For this review, take the finished solid that the model builds, in its own axes (mm). A direction names the side the tool comes from. Coordinates: 2 decimals unless noted, no trailing zeros. Write each loop counter-clockwise with the first axis right and the second up, starting at its lowest first coordinate (ties: lowest second). Pieces come first, ordered by that corner, then holes. Notation, with made-up numbers: (-38, -25) -> (11, -25) arc R20 ccw to (11, 8) -> close; hole circle Ø11 at (56.5, 50). An arc over 180 degrees is marked (long way). Put each result on its own line as item: value. Start each with the question number.
Item 1: Insertion check: P1, Ø4, axis at x = -12.73, y = -30.38, coming from the +Z side; P2, Ø2, axis at x = -10.5, y = 22, coming from the +Z side; P3, Ø1, axis at y = 15.5, z = 10, coming from the +X side; P4, Ø9.5, axis at x = -2.5, y = -13, coming from the -Z side. Each pin has a flat end and moves straight along its axis. Give the tip position at first contact, or say it passes through.
Item 2: For faces 1 (the flat face through (-4, 22.359, 1)), 2 (the flat face through (-15, -30, 0)), 3 (the flat face through (7, -30, 0)), 4 (the cylindrical face through (12.01, -26.95, -1.52)), 5 (the cylindrical face through (-19.464, 22.929, -1.521)), list the 3-axis set-ups (+Z, -Z, +X, -X, +Y, -Y) from which the entire face can be reached by the end or side of a thin tool; tool diameter is ignored.
Item 3: Consider section D-D on y = -27. Give the boundary of the cut face in (x, z).
Item 4: Consider section B-B on x = 7.5. Give the boundary of the cut face in (y, z).
Item 5: To check wall thickness, follow L1, parallel to Y at x = -5.5, z = -1.5; L2, parallel to X at y = -29.5, z = 6; L3, parallel to Z at x = -9, y = -3. State the ranges of each line that lie inside material, in increasing order.
Item 6: Consider section C-C on z = -1.5. Give the boundary of the cut face in (x, y).
Item 7: Consider section A-A on z = 6. Give the boundary of the cut face in (x, y).
Item 8: The part is to be moulded in two halves that separate along Y. For faces 6 (the flat face through (-4, -2, 10)), 7 (the cylindrical face through (12.01, -33.81, -1.52)), 8 (the flat face through (-4, 26, -3)), say which applies: +Y half, -Y half, draft (parallel to the pull), parting line (faces both ways), or undercut.
```python
from build123d import *

# Parameters (mm, degrees)
SKETCH_1_W             = 32.677388302
SKETCH_1_H             = 8
EXTRUDE_1_DEPTH        = 3
SKETCH_2_R             = 1.5
CUT_EXTRUDE_1_DEPTH    = 4
SKETCH_3_R             = 6
EXTRUDE_2_DEPTH        = 8
EXTRUDE_3_DEPTH        = 8
SKETCH_10_W            = 12
SKETCH_10_H            = 24.37
EXTRUDE_5_DEPTH        = 2
SKETCH_4_R             = 4
CUT_EXTRUDE_2_DEPTH    = 9
FILLET_1_R             = 2
MIRROR_3_COPY_1_DEPTH  = 8
FILLET_1_OF_MIRROR_3_R = 2


with BuildPart() as part:
    # Sketch 1 → Extrude 1 (new body)
    with BuildSketch(Plane.XY):
        with Locations((-3.726697353, 26.358574689)):
            Rectangle(SKETCH_1_W, SKETCH_1_H)
    extrude_1 = extrude(amount=-EXTRUDE_1_DEPTH)

    # Sketch 2 → Cut-Extrude 1 (cut, through all)
    with BuildSketch(Plane.XY):
        with Locations((-12.726697353, 26.358574689)):
            Circle(SKETCH_2_R)
        with Locations((5.273302647, 26.358574689)):
            Circle(SKETCH_2_R)
    cut_extrude_1 = extrude(amount=-CUT_EXTRUDE_1_DEPTH, mode=Mode.SUBTRACT)



with BuildPart() as body_2:
    # Sketch 3 → Extrude 2 (new body)
    with BuildSketch(Plane.XZ.offset(-22.358574689)):
        with Locations((-3.726697353, 6)):
            Circle(SKETCH_3_R)
    extrude_2 = extrude(amount=-EXTRUDE_2_DEPTH)


with BuildPart() as part_1:
    add(part.part)

    add(body_2.part)  # Extrude 3 merges body 2
    # Sketch 5 → Extrude 3 (add)
    with BuildSketch(Plane.XZ.offset(-22.358574689)):
        Polygon((-3.726697353, 0), (-9.726697353, 6), (-9.726697353, 0), align=None)
        Polygon((2.273302647, 6), (-3.726697353, 0), (2.273302647, 0), align=None)
    extrude_3 = extrude(amount=-EXTRUDE_3_DEPTH)

    # Mirror 1: Extrude 3 across plane
    add(extrude_3.mirror(Plane(origin=(0, 0, 6), x_dir=(1, 0, 0), z_dir=(0, 0, -1))))

    # Sketch 10 → Extrude 5 (add)
    with BuildSketch(Plane.XY.offset(12)):
        with Locations((-3.726697353, 10.173574689)):
            Rectangle(SKETCH_10_W, SKETCH_10_H)
    extrude_5 = extrude(amount=-EXTRUDE_5_DEPTH)

    # Sketch 4 → Cut-Extrude 2 (cut, through all)
    with BuildSketch(Plane.XZ.offset(-22.358574689)):
        with Locations((-3.726697353, 6)):
            Circle(SKETCH_4_R)
    cut_extrude_2 = extrude(amount=-CUT_EXTRUDE_2_DEPTH, mode=Mode.SUBTRACT)

    # Fillet 1
    fillet_1_edges = [part_1.edges().sort_by_distance(p)[0] for p in [
        (12.611996798, 22.358574689, -1.5),
        (-20.065391504, 22.358574689, -1.5),
        (-20.065391504, 30.358574689, -1.5),
        (12.611996798, 30.358574689, -1.5),
    ]]
    fillet(fillet_1_edges, radius=FILLET_1_R)

    # Mirror 3: Extrude 1, Cut-Extrude 1, Extrude 2, Cut-Extrude 2, Extrude 3, Extrude 5 across plane
    add(extrude_1.mirror(Plane(origin=(-9.726697353, -2.011425311, 10), x_dir=(0, 0, 1), z_dir=(0, -1, 0))))
    add(cut_extrude_1.mirror(Plane(origin=(-9.726697353, -2.011425311, 10), x_dir=(0, 0, 1), z_dir=(0, -1, 0))), mode=Mode.SUBTRACT)
    add(extrude_2.mirror(Plane(origin=(-9.726697353, -2.011425311, 10), x_dir=(0, 0, 1), z_dir=(0, -1, 0))))
    add(cut_extrude_2.mirror(Plane(origin=(-9.726697353, -2.011425311, 10), x_dir=(0, 0, 1), z_dir=(0, -1, 0))), mode=Mode.SUBTRACT)
    add(extrude_3.mirror(Plane(origin=(-9.726697353, -2.011425311, 10), x_dir=(0, 0, 1), z_dir=(0, -1, 0))))
    add(extrude_5.mirror(Plane(origin=(-9.726697353, -2.011425311, 10), x_dir=(0, 0, 1), z_dir=(0, -1, 0))))

    # Mirror 3 copy 1 sketch → Mirror 3 copy 1 (add)
    with BuildSketch(Plane(origin=(0, -26.381425311, 12), x_dir=(1, 0, 0), z_dir=(0, 1, 0))):
        Polygon((-3.726697353, 0), (-9.726697353, 6), (-9.726697353, 0), align=None)
        Polygon((2.273302647, 6), (-3.726697353, 0), (2.273302647, 0), align=None)
    extrude(amount=-MIRROR_3_COPY_1_DEPTH)

    # Fillet 1 of Mirror 3
    fillet_1_of_mirror_3_edges = [part_1.edges().sort_by_distance(p)[0] for p in [
        (12.611996798, -26.381425311, -1.5),
        (-20.065391504, -26.381425311, -1.5),
        (-20.065391504, -34.381425311, -1.5),
        (12.611996798, -34.381425311, -1.5),
    ]]
    fillet(fillet_1_of_mirror_3_edges, radius=FILLET_1_OF_MIRROR_3_R)


solid = part_1.part
```
Return value:
1. P1: z = 0
1. P2: z = 12
1. P3: x = 2.27
1. P4: z = 10
2. face 1: -Z, +X, -X
2. face 2: +Z, -X, +Y, -Y
2. face 3: +Z, +X, +Y, -Y
2. face 4: +Z, -Z, +X
2. face 5: +Z, -Z, -X
3. outline: (-19.51, -3) -> (12.06, -3) -> (12.06, 0) -> (2.27, 0) -> (2.27, 12) -> (-9.73, 12) -> (-9.73, 0) -> (-19.51, 0) -> close; hole circle Ø8 at (-3.73, 6)
4. outline: (-34.38, -3) -> (-26.38, -3) -> (-26.38, 0) -> (-34.38, 0) -> close; (22.36, -3) -> (30.36, -3) -> (30.36, 0) -> (22.36, 0) -> close
5. L1: -34.38 to -26.38, 22.36 to 30.36
5. L2: -9.73 to -7.73, 0.27 to 2.27
5. L3: 10 to 12
6. outline: (-20.07, -32.38) arc R2 ccw to (-18.07, -34.38) -> (10.61, -34.38) arc R2 ccw to (12.61, -32.38) -> (12.61, -28.38) arc R2 ccw to (10.61, -26.38) -> (-18.07, -26.38) arc R2 ccw to (-20.07, -28.38) -> close; (-20.07, 24.36) arc R2 ccw to (-18.07, 22.36) -> (10.61, 22.36) arc R2 ccw to (12.61, 24.36) -> (12.61, 28.36) arc R2 ccw to (10.61, 30.36) -> (-18.07, 30.36) arc R2 ccw to (-20.07, 28.36) -> close; hole circle Ø3 at (-12.73, -30.38); hole circle Ø3 at (-12.73, 26.36); hole circle Ø3 at (5.27, -30.38); hole circle Ø3 at (5.27, 26.36)
7. outline: (-9.73, -34.38) -> (-7.73, -34.38) -> (-7.73, -26.38) -> (-9.73, -26.38) -> close; (-9.73, 22.36) -> (-7.73, 22.36) -> (-7.73, 30.36) -> (-9.73, 30.36) -> close; (0.27, -34.38) -> (2.27, -34.38) -> (2.27, -26.38) -> (0.27, -26.38) -> close; (0.27, 22.36) -> (2.27, 22.36) -> (2.27, 30.36) -> (0.27, 30.36) -> close
8. face 6: undercut
8. face 7: -Y half
8. face 8: draft
